Can you work these out from the drawing? Everything is in mm from the part's minimum corner. A direction names the side the tool comes from. Round coordinates to 2 decimals unless told otherwise and drop trailing zeros. Write each loop counter-clockwise with the first axis right and the second up, starting at its lowest first coordinate (ties: lowest second). Pieces come first, ordered by that corner, then holes. Notation, with made-up numbers: (50.25, -27) -> (56.25, -27) arc R28 ccw to (56.25, 9) -> close; hole circle Ø9 at (-36, 36). An arc over 180 degrees is marked (long way). Answer as CSV lines item,"result". Start each with the question number.
Q1. If I drill on line 1 (Z direction, x = 15, y = 1.05); line 2 (X direction, y = 1, z = 7.5); line 3 (Y direction, x = 18.5, z = 5) (1 decimal), over which ranges is the centre line in solid material (lowest first)? Write a range as [from, to].
Q2. For the marked faces 4, 5 and 6, which set-ups out of +Z, -Z, +X, -X, +Y, -Y let a thin tool reach every point of the face, with its end or its side?
Q3. Imagine slicing it at C-C on y = 48.5. Please give me the cut outline in (x, z).
Q4. Imagine slicing it at A-A on x = 15. Please give me the cut outline in (y, z) (1 decimal).
Q5. Will these pins go through, and if not, where does the flat tip stop? pin 1 Ø3 at (x, z) = (9, 7) entering from +Y; pin 2 Ø1.5 at (x, z) = (23, 10) entering from -Y.
Q6. Imagine slicing it at B-B on z = 3. Please give me the cut outline in (x, y) (1 decimal).
Q7. If we mould it in two halves opening along X, with no side actions, what happens to the marked faces 1, 2 and 3? For each: pulls with the +X half, pulls with the -X half, needs draft (parallel to the pull), parting line crosses it, or undercut.
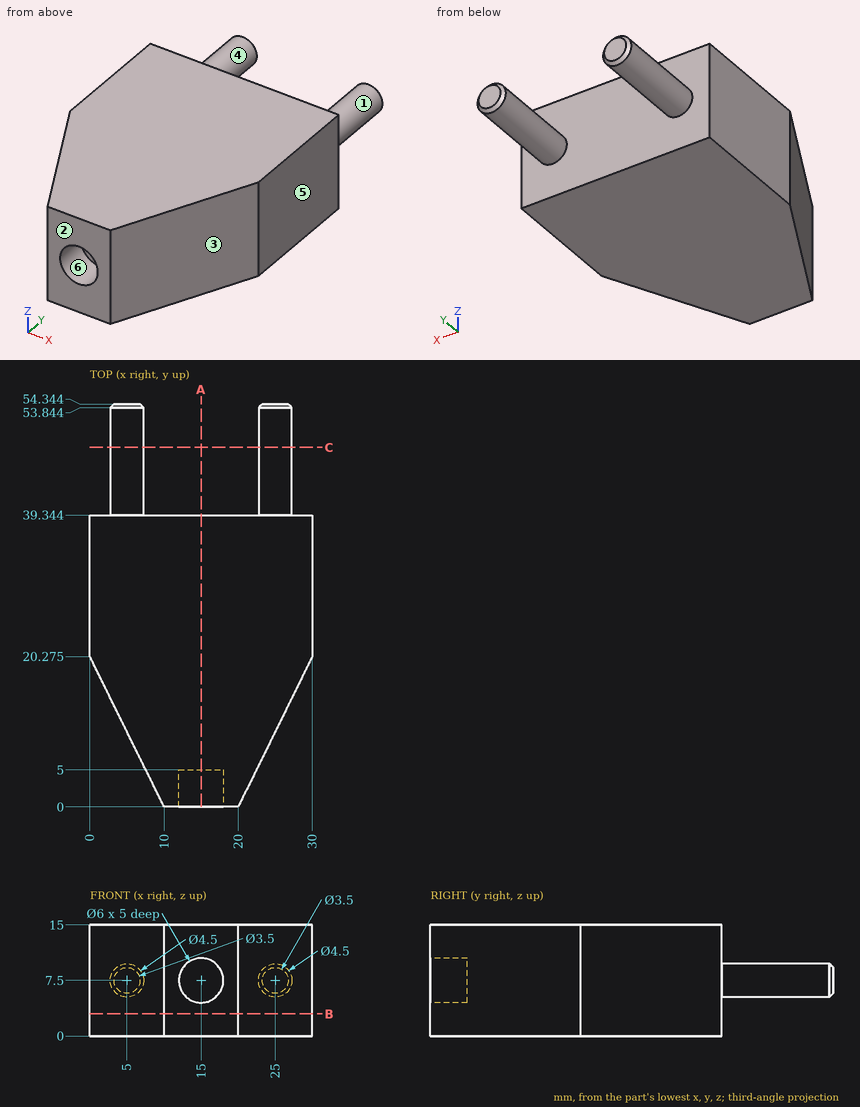
Checks:
1,line 1,"[0, 4.5], [10.5, 15]"
1,line 2,"[9.51, 12], [18, 20.49]"
1,line 3,"[0, 39.3]"
2,face 4,"+Y"
2,face 5,"+Z, -Z, +X, +Y, -Y"
2,face 6,"-Y"
3,outline,"circle Ø4.5 at (5, 7.5); circle Ø4.5 at (25, 7.5)"
4,outline,"(0, 0) -> (39.3, 0) -> (39.3, 15) -> (0, 15) -> (0, 10.5) -> (5, 10.5) -> (5, 4.5) -> (0, 4.5) -> close"
5,pin 1,"y = 39.34"
5,pin 2,"y = 4.56"
6,outline,"(0, 20.3) -> (10, 0) -> (20, 0) -> (30, 20.3) -> (30, 39.3) -> (0, 39.3) -> close"
7,face 1,"undercut"
7,face 2,"needs draft"
7,face 3,"pulls with the +X half"
